Check sheet for the modelled part. Datum: model origin and axes. Units: mm. A direction names the side the tool comes from. Round coordinates to 2 decimals unless told otherwise and drop trailing zeros. Write each loop counter-clockwise with the first axis right and the second up, starting at its lowest first coordinate (ties: lowest second). Pieces come first, ordered by that corner, then holes.
Item 1: Release check for a two-part mould opening along Z. For faces 4 (the flat face through (-40.2, 6.9, 0)), 5 (the cylindrical face through (-15.241, -58.905, 21.316)), 6 (the flat face through (-1, 45, 11)) record: pulls with the +Z half, pulls with the -Z half, needs draft (parallel to the pull), parting line crosses it, or undercut.
Item 2: Section check B-B, the plane y = -12.5. Record the cut outline in (x, z), plus the area to 3 significant figures.
Item 3: Section check A-A, the plane x = 0. Record the cut outline in (y, z).
Item 4: Set-up check for faces 1 (the cylindrical face through (-15.258, -67.497, 20.724)), 2 (the flat face through (-40, -1, 20)), 3 (the flat face through (45, -1, 20)): record each of +Z, -Z, +X, -X, +Y, -Y from which the full face is reachable in a straight line by a thin tool's end or side.
Item 5: Depth check by flat-ended pin: pin 1 (6 mm diameter, centred on y = -53, z = 18.5, fed in from -X); pin 2 (19 mm diameter, centred on x = 0, z = 20, fed in from -Y). Enter the tip coordinate at first touch or a pass-through.
Item 6: Section check D-D, the plane z = 20. State how many separate pieces and enclosed holes the cut face has, plus the area to 3 significant figures.
Item 7: Material ranges on line 1 along Y through (x, z) = (15.5, 20); line 2 along X through (y, z) = (-20, 8.5); line 3 along X through (y, z) = (41.3, 20), recorded low to high.
from build123d import *

# Parameters (mm, degrees)
SKETCH_1_W           = 90
SKETCH_1_H           = 90
SKETCH_1_W_2         = 80
SKETCH_1_H_2         = 80
EXTRUDE_1_DEPTH      = 40
SKETCH_3_R           = 6
CUT_EXTRUDE_2_DEPTH  = 109.282039139
EXTRUDE_2_DEPTH      = 20
EXTRUDE_2_DEPTH_BACK = 20
SKETCH_4_R           = 4
SKETCH_5_W           = 22
SKETCH_5_H           = 30
CUT_EXTRUDE_3_DEPTH  = 88.510910897


with BuildPart() as part:
    # Sketch 1 → Extrude 1 (new body)
    with BuildSketch(Plane.XY):
        Rectangle(SKETCH_1_W, SKETCH_1_H)
        Rectangle(SKETCH_1_W_2, SKETCH_1_H_2, mode=Mode.SUBTRACT)
    extrude(amount=EXTRUDE_1_DEPTH)

    # Sketch 3 → Cut-Extrude 2 (cut, through all)
    with BuildSketch(Plane(origin=(0, 45, 0), x_dir=(1, 0, 0), z_dir=(0, 1, 0))):
        with Locations(Location((0, -20, 0), (0, 0, 270))):
            Circle(SKETCH_3_R)
    extrude(amount=-CUT_EXTRUDE_2_DEPTH, mode=Mode.SUBTRACT)

    # Sketch 4 → Extrude 2 (add, two sides: drawn at the far end of the back side and taken through both)
    with BuildSketch(Plane(origin=(1.596612883, -1.997656421, 74.241754421), x_dir=(-0.029422382723106603, 0, -0.9995670679823816), z_dir=(0.9995670679823816, 0, -0.029422382723106603)).offset(-EXTRUDE_2_DEPTH_BACK)):
        with BuildLine():
            Line((41.765247584, -43.002343579), (41.765247584, -53.002343579))
            ThreePointArc((41.765247584, -53.002343579), (54.265247584, -65.502343579), (66.765247584, -53.002343579))
            Line((66.765247584, -53.002343579), (66.765247584, -43.002343579))
            Line((66.765247584, -43.002343579), (41.765247584, -43.002343579))
        make_face()
        with Locations((54.265247584, -53.002343579)):
            Circle(SKETCH_4_R, mode=Mode.SUBTRACT)
    extrude(amount=EXTRUDE_2_DEPTH + EXTRUDE_2_DEPTH_BACK)

    # Sketch 5 → Cut-Extrude 3 (cut, through all)
    with BuildSketch(Plane(origin=(0.220413113, 0, 7.488098118), x_dir=(-0.9995670679823816, 0, 0.0294223827231066), z_dir=(-0.0294223827231066, 0, -0.9995670679823816))):
        with Locations((0, -60)):
            Rectangle(SKETCH_5_W, SKETCH_5_H)
    extrude(amount=-CUT_EXTRUDE_3_DEPTH, mode=Mode.SUBTRACT)


solid = part.part
Values found:
1. face 4: pulls with the -Z half
1. face 5: undercut
1. face 6: needs draft
2. outline: (-45, 0) - (-40, 0) - (-40, 40) - (-45, 40) - close; (40, 0) - (45, 0) - (45, 40) - (40, 40) - close
2. area: 400 mm2
3. outline: (-45, 0) - (-40, 0) - (-40, 14) - (-45, 14) - close; (-45, 26) - (-40, 26) - (-40, 40) - (-45, 40) - close; (40, 0) - (45, 0) - (45, 14) - (40, 14) - close; (40, 26) - (45, 26) - (45, 40) - (40, 40) - close
4. face 1: -Y
4. face 2: +Z, -Z
4. face 3: +Z, -Z, +X, +Y, -Y
5. pin 1: stops at x = -20.14
5. pin 2: stops at y = -45
6. separate pieces: 4
6. enclosed holes: 0
6. area: 1,840 mm2
7. line 1: y = -67.49 to -58.97, -51.03 to -40, 40 to 45
7. line 2: x = -45 to -40, 40 to 45
7. line 3: x = -45 to -6, 6 to 45
